Source: CAD feature listing. Evaluate the final solid. Frame: model axes, mm. Face numbers are marked on the shaded views. Coordinates: 2 decimals unless noted, no trailing zeros. Write each loop counter-clockwise with the first axis right and the second up, starting at its lowest first coordinate (ties: lowest second). Pieces come first, ordered by that corner, then holes. Notation, with made-up numbers: (45.5, 88.5) -> (62.5, 88.5) arc R9 cw to (62.5, 102.5) -> close; hole circle Ø3 at (-8, 5). An arc over 180 degrees is marked (long way). One line per item, written item: value. Start each with the question number.
1. Section query D-D, the plane x = 15. Output: boundary loops of the cut face in (y, z).
2. Section query C-C, the plane y = 16.25. Output: boundary loops of the cut face in (x, z).
3. Mould query, pull axis Y, two halves, no side actions, for the marked faces 1 and 2. Classes: released by +Y, released by -Y, zero draft, split by the parting line, or undercut.
4. Section query A-A, the plane z = -315.5. Output: boundary loops of the cut face in (x, y).
5. Section query B-B, the plane z = -98. Output: boundary loops of the cut face in (x, y).
6. First-contact query: P1, Ø8.5, axis at x = -60.86, z = -173.79, coming from the +Y side; P2, Ø10.5, axis at x = -87.53, z = -173.79, coming from the -Y side; P3, Ø2, axis at y = 3, z = -289.5, coming from the +X side; P4, Ø1.4, axis at x = -111.5, y = 11, coming from the +Z side. Flat tips, straight axial feed; report the tip coordinate or a pass-through.
7. Line query: line 1 (Y direction, x = 85, z = -221.5); line 2 (X direction, y = 7.75, z = -224). Output: solid intervals per line, ascending.
from build123d import *

# Parameters (mm, degrees)
SKETCH1_R                     = 7.9375
SKETCH1_R_2                   = 3.302
BASE_FLANGE1_DEPTH            = 2.54
EDGE_FLANGE1_STRIP_W          = 11.6332
EDGE_FLANGE1_STRIP_H          = 2.54
EDGE_FLANGE1_STRIP_CUT_DEPTH  = 308.6735
EDGE_FLANGE1_RELIEF_W         = 12.9032
EDGE_FLANGE1_RELIEF_H         = 1.27
EDGE_FLANGE1_RELIEF_CUT_DEPTH = 2.54
EDGE_FLANGE1_DEPTH            = 308.6735


# Sheet-metal steps are written as plain solids
with BuildPart() as part:
    # Sketch1 → Base-Flange1 (new body)
    with BuildSketch(Plane(origin=(0, 0, 0), x_dir=(1, 0, 0), z_dir=(0, 1, 0))):
        with BuildLine():
            Line((109.619528436, 311.807263764), (89.361961148, 247.115522342))
            ThreePointArc((89.361961148, 247.115522342), (89.460566801, 224.034337943), (102.867006006, 205.245559798))
            ThreePointArc((102.867006006, 205.245559798), (108.478001121, 198.524407286), (110.49, 190.003314763))
            Line((110.49, 190.003314763), (110.49, 0))
            Line((110.49, 0), (-114.3, 0))
            Line((-114.3, 0), (-114.3, 336.55))
            Line((-114.3, 336.55), (-67.202083301, 336.55))
            ThreePointArc((-67.202083301, 336.55), (0, 311.15), (67.202083301, 336.55))
            Line((67.202083301, 336.55), (91.44, 336.55))
            ThreePointArc((91.44, 336.55), (106.791695758, 328.779536221), (109.619528436, 311.807263764))
        make_face()
        with Locations(Location((-86.36, 317.5, 0), (0, 0, 270))):
            Circle(SKETCH1_R, mode=Mode.SUBTRACT)
        with Locations(Location((91.44, 317.5, 0), (0, 0, 270))):
            Circle(SKETCH1_R, mode=Mode.SUBTRACT)
        with Locations(Location((91.44, 190.003314763, 0), (0, 0, 270))):
            Circle(SKETCH1_R, mode=Mode.SUBTRACT)
        with Locations(Location((-86.36, 77.503314763, 0), (0, 0, 270))):
            Circle(SKETCH1_R, mode=Mode.SUBTRACT)
        with Locations(Location((-60.8584, 173.787563647, 0), (0, 0, 270))):
            Circle(SKETCH1_R_2, mode=Mode.SUBTRACT)
        with Locations(Location((-87.5284, 173.787563647, 0), (0, 0, 270))):
            Circle(SKETCH1_R_2, mode=Mode.SUBTRACT)
        with Locations(Location((-60.8584, 117.145563647, 0), (0, 0, 270))):
            Circle(SKETCH1_R_2, mode=Mode.SUBTRACT)
        with Locations(Location((-87.5284, 117.145563647, 0), (0, 0, 270))):
            Circle(SKETCH1_R_2, mode=Mode.SUBTRACT)
    extrude(amount=-BASE_FLANGE1_DEPTH)

    # Edge-Flange1 strip (across the edge) → Edge-Flange1 strip cut (cut)
    with BuildSketch(Plane(origin=(-114.3, 0, -336.55), x_dir=(1, 0, 0), z_dir=(0, 0, 1))):
        with Locations((-2.54, -1.27)):
            Rectangle(EDGE_FLANGE1_STRIP_W, EDGE_FLANGE1_STRIP_H)
    extrude(amount=EDGE_FLANGE1_STRIP_CUT_DEPTH, mode=Mode.SUBTRACT)

    # Edge-Flange1 relief (on the sheet) → Edge-Flange1 relief cut (cut)
    with BuildSketch(Plane(origin=(-111.0234, 0, -336.55), x_dir=(1, 0, 0), z_dir=(0, 1, 0))):
        with Locations((-5.1816, -309.3085)):
            Rectangle(EDGE_FLANGE1_RELIEF_W, EDGE_FLANGE1_RELIEF_H)
    extrude(amount=-EDGE_FLANGE1_RELIEF_CUT_DEPTH, mode=Mode.SUBTRACT)

    # Edge-Flange1 section (across the edge) → Edge-Flange1 (add)
    with BuildSketch(Plane(origin=(-114.3, 0, -336.55), x_dir=(1, 0, 0), z_dir=(0, 0, 1))):
        with BuildLine():
            Line((0, 0.7366), (0, 25.4))
            Line((0, 25.4), (2.54, 25.4))
            Line((2.54, 25.4), (2.54, 0.7366))
            ThreePointArc((2.54, 0.7366), (2.755745145, 0.215745145), (3.2766, 0))
            Line((3.2766, 0), (3.2766, -2.54))
            ThreePointArc((3.2766, -2.54), (0.959693921, -1.580306079), (0, 0.7366))
        make_face()
    extrude(amount=EDGE_FLANGE1_DEPTH)


solid = part.part
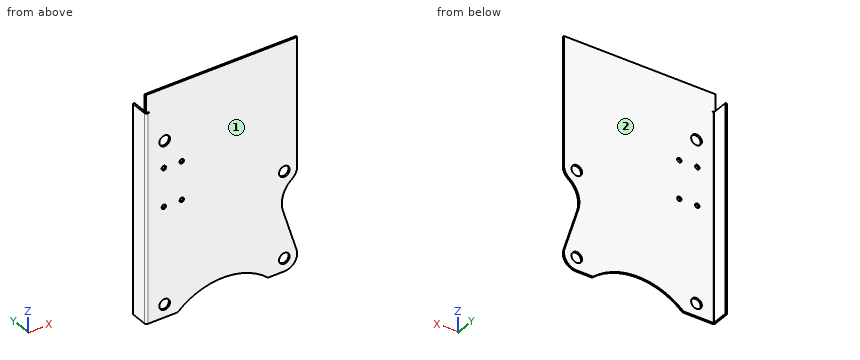
Computed values:
1. outline: (-2.54, -312.26) -> (0, -312.26) -> (0, 0) -> (-2.54, 0) -> close
2. outline: (-114.3, -336.55) -> (-111.76, -336.55) -> (-111.76, -27.88) -> (-114.3, -27.88) -> close
3. face 1: released by -Y
3. face 2: released by +Y
4. outline: (-114.3, 0.74) arc R3.28 ccw to (-111.02, -2.54) -> (-94.04, -2.54) -> (-94.04, 0) -> (-111.02, 0) arc R0.74 cw to (-111.76, 0.74) -> (-111.76, 25.4) -> (-114.3, 25.4) -> close; (-78.68, -2.54) -> (-29.41, -2.54) -> (-29.41, 0) -> (-78.68, 0) -> close; (29.41, -2.54) -> (83.76, -2.54) -> (83.76, 0) -> (29.41, 0) -> close; (99.12, -2.54) -> (110.38, -2.54) -> (110.38, 0) -> (99.12, 0) -> close
5. outline: (-114.3, 0.74) arc R3.28 ccw to (-111.02, -2.54) -> (110.49, -2.54) -> (110.49, 0) -> (-111.02, 0) arc R0.74 cw to (-111.76, 0.74) -> (-111.76, 25.4) -> (-114.3, 25.4) -> close
6. P1: stops at y = 0
6. P2: stops at y = -2.54
6. P3: stops at x = -111.76
6. P4: stops at z = -27.88
7. line 1: y = -2.54 to 0
7. line 2: x = -114.3 to -111.76
